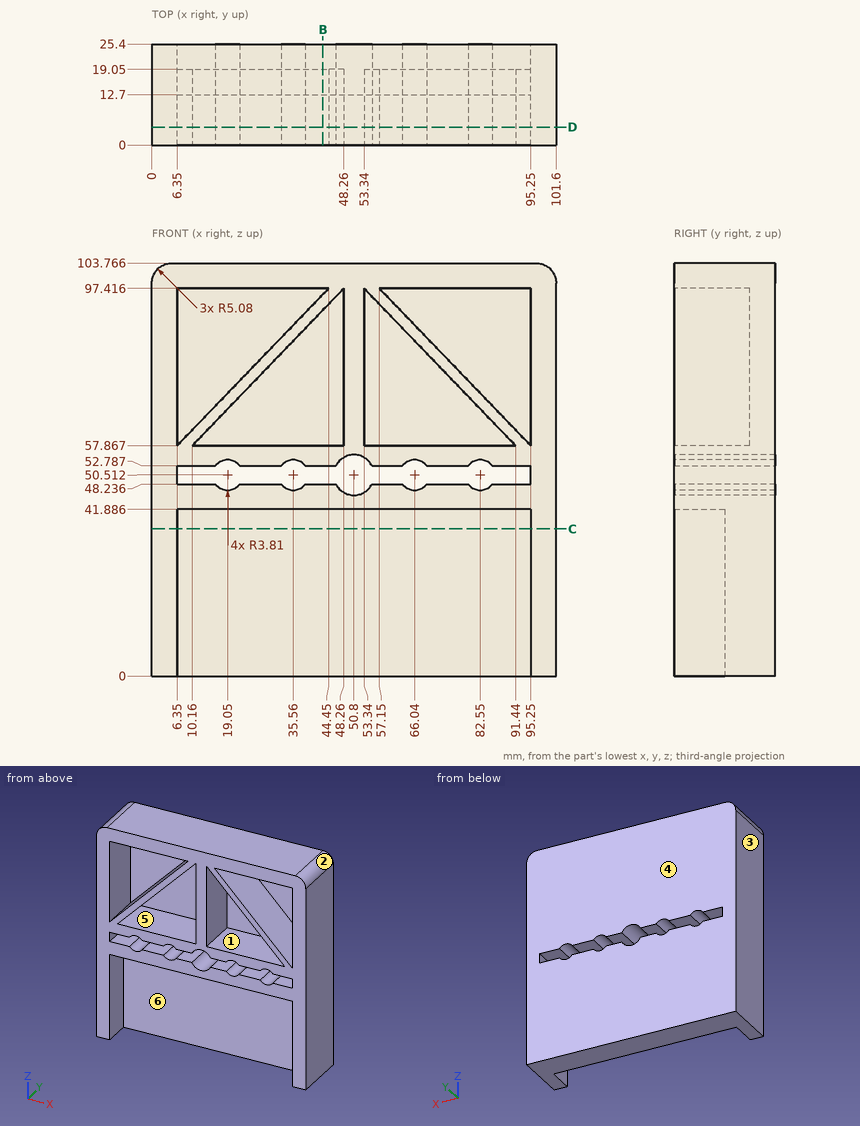
Study the drawing (mm; zero at the part's minimum x, y, z) and answer. A direction names the side the tool comes from. Round coordinates to 2 decimals unless told otherwise and drop trailing zeros. Order: outer loops, then holes, each group sorted by start corner. A loop starts at its lowest first (then second) coordinate and runs counter-clockwise, first axis right, second up. Notation, with made-up numbers: (-8.75, 8.25) - (26.25, 8.25) arc R33 ccw to (26.25, 42.25) - close; hole circle Ø1 at (46, -13). An arc over 180 degrees is marked (long way). Use one line per item in the form item = value. Start each with the question number.
(1) Find the intervals of material crossed by line 1 along X through (y, z) = (7.75, 76.5); line 2 along Z through (x, y) = (93.5, 7.75) (1 decimal); line 3 along X through (y, z) = (1, 14.5), in increasing order. Write a range as from..to.
(2) Flat-ended cylindrical pins translate along their axes: pin 1 Ø3 at (x, y) = (78, 7) entering from -Z; pin 2 Ø11.5 at (x, z) = (63.5, 83) entering from -Y; pin 3 Ø21 at (x, z) = (35, 30.5) entering from -Y. Find the tip coordinate at first contact, or state that the pin passes through.
(3) Determine the mould class of the marked faces 1, 2 and 3 for opening direction X: +X half, -X half, draft (parallel to the pull), parting line (faces both ways), or undercut.
(4) The part is cut by section C-C (z = 37). Give the vertices of the cut face in (x, y), then the cut area to 3 significant figures.
(5) The part is cut by section B-B (x = 43). Give the vertices of the cut face in (y, z).
(6) For the marked faces 4, 5 and 6, determine the directions among +Z, -Z, +X, -X, +Y, -Y from which every point of the face is accessible in a straight line to the end or side of a thin tool.
(7) The part is cut by section D-D (y = 4.5). Count the separate pieces of the cut face and the enclosed holes in it, then the cut area to 3 significant figures.
Checked values:
q1.line_1 = 0..6.35, 24.3..28.11, 48.26..53.34, 73.49..77.3, 95.25..101.6
q1.line_2 = 41.9..48.2, 52.8..59.7, 97.4..103.8
q1.line_3 = 0..6.35, 95.25..101.6
q2.pin_1 = 41.89
q2.pin_2 = 0
q2.pin_3 = 12.7
q3.face_1 = undercut
q3.face_2 = +X half
q3.face_3 = -X half
q4.outline = (0, 0) - (6.35, 0) - (6.35, 12.7) - (95.25, 12.7) - (95.25, 0) - (101.6, 0) - (101.6, 25.4) - (0, 25.4) - close
q4.area = 1,450 mm^2
q5.outline = (0, 41.89) - (12.7, 41.89) - (12.7, 0) - (25.4, 0) - (25.4, 48.24) - (0, 48.24) - close; (0, 52.79) - (25.4, 52.79) - (25.4, 103.77) - (0, 103.77) - (0, 97.42) - (19.05, 97.42) - (19.05, 95.91) - (0, 95.91) - (0, 91.96) - (19.05, 91.96) - (19.05, 57.87) - (0, 57.87) - close
q6.face_4 = +Z, -Z, +X, -X, +Y
q6.face_5 = -Y
q6.face_6 = -Z, -Y
q7.separate_pieces = 1
q7.enclosed_holes = 5
q7.area = 3,300 mm^2
